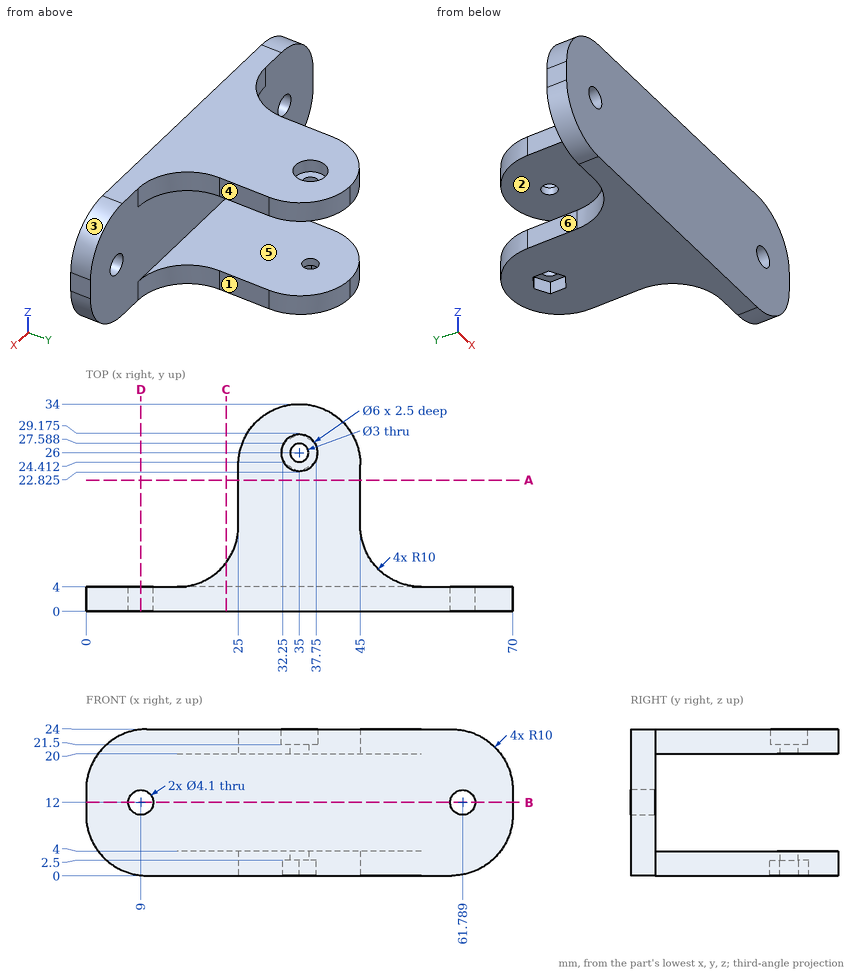
Study the drawing (mm; zero at the part's minimum x, y, z) and answer. A direction names the side the tool comes from. Coordinates: 2 decimals unless noted, no trailing zeros. Loops run counter-clockwise (first coordinate to the right, second up) from the corner with the lowest first, then second, coordinate; pieces in that order, holes last. Notation, with made-up numbers: (-27, 33) -> (23, 33) arc R32 ccw to (23, 60) -> close; hole circle Ø10 at (-26, -12). An arc over 180 degrees is marked (long way). Answer as CSV lines item,"result".
1) The part is cut by section A-A (y = 21.5). Give the vertices of the cut face in (x, z), and give its area (3 significant figures).
A:
outline,"(25, 0) -> (45, 0) -> (45, 4) -> (25, 4) -> close; (25, 20) -> (45, 20) -> (45, 24) -> (25, 24) -> close"
area,"160 mm²"
2) The part is cut by section D-D (x = 9). Give the vertices of the cut face in (y, z), and give its area (3 significant figures).
A:
outline,"(0, 0.05) -> (4, 0.05) -> (4, 9.95) -> (0, 9.95) -> close; (0, 14.05) -> (4, 14.05) -> (4, 23.95) -> (0, 23.95) -> close"
area,"79.2 mm²"
3) The part is cut by section B-B (z = 12). Give the vertices of the cut face in (x, y), and give its area (3 significant figures).
A:
outline,"(0, 0) -> (6.95, 0) -> (6.95, 4) -> (0, 4) -> close; (11.05, 0) -> (59.74, 0) -> (59.74, 4) -> (11.05, 4) -> close; (63.84, 0) -> (70, 0) -> (70, 4) -> (63.84, 4) -> close"
area,"247 mm²"
4) For a pull along Z with two mould halves and no side action, classify the marked faces 1, 2 and 3 as released by +Z, released by -Z, zero draft, split by the parting line, or undercut.
A:
face 1,"zero draft"
face 2,"undercut"
face 3,"released by +Z"
5) For the marked faces 4, 5 and 6, determine the directions among +Z, -Z, +X, -X, +Y, -Y from which every point of the face is accessible in a straight line to the end or side of a thin tool.
A:
face 4,"+Z, -Z, +X, +Y"
face 5,"+X, -X, +Y"
face 6,"+Z, -Z, -X, +Y"
6) Flat-ended cylindrical pins translate along their axes: pin 1 (3 mm diameter, centred on x = 59, z = 7.5, fed in from +Y); pin 2 (8 mm diameter, centred on y = 16, z = 10.5, fed in from -X); pin 3 (2 mm diameter, centred on y = 18.5, z = 21, fed in from -X); pin 4 (3.5 mm diameter, centred on x = 35, y = 26, fed in from +Z). Find the tip coordinate at first contact, or state that the pin passes through.
A:
pin 1,"stops at y = 4"
pin 2,"passes through"
pin 3,"stops at x = 25"
pin 4,"stops at z = 21.5"
7) The part is cut by section C-C (x = 23). Give the vertices of the cut face in (y, z).
A:
outline,"(0, 0) -> (8, 0) -> (8, 4) -> (4, 4) -> (4, 20) -> (8, 20) -> (8, 24) -> (0, 24) -> close"
8) Straight lines are drawn through the part: probe 1 along X at (y, z) = (0.85, 12); probe 2 along X at (y, z) = (2, 13.25) (1 decimal); probe 3 along Z at (x, y) = (31, 6). For each, find the intervals that lie inside material, in ascending order.
A:
probe 1,"x = 0 to 6.95, 11.05 to 59.74, 63.84 to 70"
probe 2,"x = 0 to 7.4, 10.6 to 60.2, 63.4 to 70"
probe 3,"z = 0 to 4, 20 to 24"
